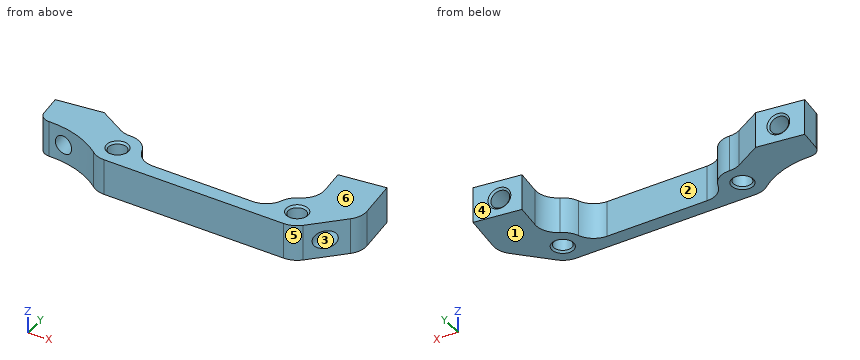
```python
from build123d import *

# Parameters (mm, degrees)
SKETCH_1_R                  = 2.5
EXTRUDE_1_DEPTH             = 10
HOLE_WIZARD_M61_AT_2_COUNT  = 2
HOLE_WIZARD_M61_AT_2_PITCH  = 51
HOLE_WIZARD_M62_D           = 5
HOLE_WIZARD_M62_CSINK_D     = 6.05
HOLE_WIZARD_M62_CSINK_ANGLE = 90


with BuildPart() as part:
    # Эскиз1 → Бобышка-Вытянуть1 (new body)
    with BuildSketch(Plane.XY):
        with BuildLine():
            Line((130.883213409, -0.667537052), (132.243357005, -11.745017689))
            ThreePointArc((132.243357005, -11.745017689), (131.983826113, -14.362626415), (130.629567818, -16.617668809))
            Line((130.629567818, -16.617668809), (122.596022679, -25.039275591))
            ThreePointArc((122.596022679, -25.039275591), (120.615825879, -26.413663696), (118.254534957, -26.897840532))
            Line((118.254534957, -26.897840532), (67.254534957, -26.897840532))
            ThreePointArc((67.254534957, -26.897840532), (65.137379079, -26.511898867), (63.292589424, -25.403724196))
            ThreePointArc((63.292589424, -25.403724196), (55.75092202, -21.419041585), (47.318028666, -20.138123004))
            ThreePointArc((47.318028666, -20.138123004), (45.29848634, -19.402158499), (44.289626193, -17.504160563))
            Line((44.289626193, -17.504160563), (43.539152064, -11.392039271))
            Line((43.539152064, -11.392039271), (56.442252036, -9.807737807))
            Line((56.442252036, -9.807737807), (63.876575818, -14.099946644))
            ThreePointArc((63.876575818, -14.099946644), (65.415135622, -14.723089071), (67.065555387, -14.900817376))
            ThreePointArc((67.065555387, -14.900817376), (70.641046717, -15.944908259), (72.911389206, -18.897840532))
            ThreePointArc((72.911389206, -18.897840532), (75.10414184, -21.796820017), (78.568243456, -22.897840532))
            Line((78.568243456, -22.897840532), (106.940826458, -22.897840532))
            ThreePointArc((106.940826458, -22.897840532), (110.404928073, -21.796820017), (112.597680707, -18.897840532))
            ThreePointArc((112.597680707, -18.897840532), (113.760800632, -16.922120242), (115.58004554, -15.526890303))
            ThreePointArc((115.58004554, -15.526890303), (118.190187148, -12.997185387), (118.860833034, -9.424724013))
            Line((118.860833034, -9.424724013), (117.980113437, -2.251838516))
            Line((117.980113437, -2.251838516), (130.883213409, -0.667537052))
        make_face()
        with Locations((67.254534957, -20.897840532)):
            Circle(SKETCH_1_R, mode=Mode.SUBTRACT)
        with Locations((118.254534957, -20.897840532)):
            Circle(SKETCH_1_R, mode=Mode.SUBTRACT)
    extrude(amount=EXTRUDE_1_DEPTH)

    # Эскиз2 → Отверстие обработанное метчиком M61 (revolve, cut)
    with BuildSketch(Plane(origin=(67.254534957, -20.897840532, 10), x_dir=(0, -1, 0), z_dir=(1, 0, 0))):
        Polygon((0, 0), (0, 10), (3.025, 10), (2.5, 9.475), (2.5, 0.525), (3.025, 0), align=None)
    hole_wizard_m61 = revolve(axis=Axis((67.254534957, -20.897840532, 16.35), (0, 0, -1)), mode=Mode.SUBTRACT)

    # Отверстие обработанное метчиком M61 at 2: Отверстие обработанное метчиком M61 ×2
    with Locations(*[(i * HOLE_WIZARD_M61_AT_2_PITCH, 0, 0) for i in range(1, HOLE_WIZARD_M61_AT_2_COUNT)]):
        add(hole_wizard_m61, mode=Mode.SUBTRACT)

    # Отверстие обработанное метчиком M62 (through all)
    with Locations(Plane(origin=(2.024641313, -16.489380245, 0), x_dir=(-0.992546151641322, -0.12186934340514836, 0), z_dir=(-0.12186934340514835, 0.9925461516413219, 0))):
        with Locations((-48.826277481, 5), (-122.826277481, 5)):
            CounterSinkHole(HOLE_WIZARD_M62_D / 2, HOLE_WIZARD_M62_CSINK_D / 2, counter_sink_angle=HOLE_WIZARD_M62_CSINK_ANGLE)


solid = part.part
```
For this review, take the finished solid that the model builds, in its own axes (mm). Face numbers are marked on the shaded views. A direction names the side the tool comes from. Coordinates: 2 decimals unless noted, no trailing zeros. Write each loop counter-clockwise with the first axis right and the second up, starting at its lowest first coordinate (ties: lowest second). Pieces come first, ordered by that corner, then holes.
(1) Tool access review of the marked faces 1 and 2: name each direction out of +Z, -Z, +X, -X, +Y, -Y from which nothing blocks a thin tool from reaching the whole face with its end or side.
(2) For pin 1 Ø5 at (x, z) = (104, 6.5) entering from +Y; pin 2 Ø4 at (y, z) = (-22.5, 1) entering from +X, all flat-tipped, find the tip position at first contact; note any pin that passes through.
(3) Wall thickness on probe 1 along Y at (x, z) = (96, 9.25); probe 2 along X at (y, z) = (-6, 5.5); probe 3 along Y at (x, z) = (67.5, 1.5): over which ranges is each line inside the solid? List them lowest first.
(4) The part is to be moulded in two halves that separate along X. For the marked faces 3, 4, 5 and 6, say which applies: +X half, -X half, draft (parallel to the pull), parting line (faces both ways), or undercut.
(5) Add section A-A on z = 6.75. Count the separate pieces of the cut face and the enclosed holes in it, then the cut area to 3 significant figures.
(6) Add section C-C on x = 83. Give the boundary of the cut face in (y, z).
Answer sheet:
1. face 1: -Z, +X, -X, +Y, -Y
1. face 2: +Z, -Z, +Y
2. pin 1: stops at y = -22.9
2. pin 2: stops at x = 126.93
3. probe 1: y = -26.9 to -22.9
3. probe 2: x = 118.44 to 122.02, 126.95 to 131.54
3. probe 3: y = -26.9 to -23.39, -18.41 to -14.9
4. face 3: undercut
4. face 4: -X half
4. face 5: +X half
4. face 6: draft
5. separate pieces: 3
5. enclosed holes: 2
5. area: 674 mm2
6. outline: (-26.9, 0) - (-22.9, 0) - (-22.9, 10) - (-26.9, 10) - close
